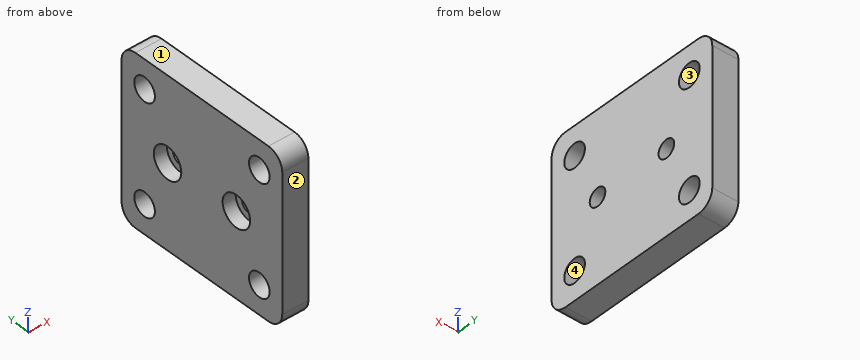
from build123d import *

# Parameters (mm, degrees)
SKETCH_1_W      = 32
SKETCH_1_H      = 35
SKETCH_1_R      = 2.25
SKETCH_1_R_2    = 3
EXTRUDE_1_DEPTH = 2.5
SKETCH_2_W      = 32
SKETCH_2_H      = 35
SKETCH_2_R      = 2.25
SKETCH_2_R_2    = 1.7
EXTRUDE_2_DEPTH = 2.5
FILLET_1_R      = 3


with BuildPart() as part:
    # 草图1 → 凸台-拉伸1 (new body)
    with BuildSketch(Plane(origin=(0, 0, 0), x_dir=(0, 0, -1), z_dir=(1, 0, 0))):
        with Locations((16, 17.5)):
            Rectangle(SKETCH_1_W, SKETCH_1_H)
        with Locations((5.5, 30)):
            Circle(SKETCH_1_R, mode=Mode.SUBTRACT)
        with Locations((26.5, 30)):
            Circle(SKETCH_1_R, mode=Mode.SUBTRACT)
        with Locations((5.5, 5)):
            Circle(SKETCH_1_R, mode=Mode.SUBTRACT)
        with Locations((26.5, 5)):
            Circle(SKETCH_1_R, mode=Mode.SUBTRACT)
        with Locations((16, 25)):
            Circle(SKETCH_1_R_2, mode=Mode.SUBTRACT)
        with Locations((16, 10)):
            Circle(SKETCH_1_R_2, mode=Mode.SUBTRACT)
    extrude(amount=EXTRUDE_1_DEPTH)

    # 草图2 → 凸台-拉伸2 (add)
    with BuildSketch(Plane(origin=(2.5, 0, 0), x_dir=(0, 0, -1), z_dir=(1, 0, 0))):
        with Locations((16, 17.5)):
            Rectangle(SKETCH_2_W, SKETCH_2_H)
        with Locations((26.5, 5)):
            Circle(SKETCH_2_R, mode=Mode.SUBTRACT)
        with Locations((5.5, 5)):
            Circle(SKETCH_2_R, mode=Mode.SUBTRACT)
        with Locations((26.5, 30)):
            Circle(SKETCH_2_R, mode=Mode.SUBTRACT)
        with Locations((5.5, 30)):
            Circle(SKETCH_2_R, mode=Mode.SUBTRACT)
        with Locations((16, 25)):
            Circle(SKETCH_2_R_2, mode=Mode.SUBTRACT)
        with Locations((16, 10)):
            Circle(SKETCH_2_R_2, mode=Mode.SUBTRACT)
    extrude(amount=EXTRUDE_2_DEPTH)

    # 圆角1
    fillet_1_edges = [part.edges().sort_by_distance(p)[0] for p in [
        (2.5, 35, 0),
        (2.5, 35, -32),
        (2.5, 0, -32),
        (2.5, 0, 0),
    ]]
    fillet(fillet_1_edges, radius=FILLET_1_R)


solid = part.part
Verification items for the finished model (mm, model axes). Face numbers are marked on the shaded views. Coordinates: 2 decimals unless noted, no trailing zeros. Loops run counter-clockwise (first coordinate to the right, second up) from the corner with the lowest first, then second, coordinate; pieces in that order, holes last. Notation, with made-up numbers: (16, 33.25) -> (66, 33.25) arc R24 cw to (66, 69.25) -> close; hole circle Ø8 at (33, 9). An arc over 180 degrees is marked (long way). Answer as a JSON object with one key per item and string values. Group by question number.
Item 1: Scan lines: probe 1 along Y at (x, z) = (1.5, -16); probe 2 along Y at (x, z) = (3.8, -16); probe 3 along X at (y, z) = (12, -14). Record each from-to range of solid material in increasing order.
Item 2: Depth check by flat-ended pin: pin 1 (3.5 mm diameter, centred on y = 5, z = -26.5, fed in from -X); pin 2 (3.5 mm diameter, centred on y = 25, z = -16, fed in from -X). Enter the tip coordinate at first touch or a pass-through.
Item 3: Sectioned sample at D-D on x = 1.85. Record the boundary of the cut face in (y, z), plus the area to 3 significant figures.
Item 4: Sectioned sample at A-A on y = 30. Record the boundary of the cut face in (x, z).
Item 5: Sectioned sample at C-C on y = 10. Record the boundary of the cut face in (x, z), plus the area to 4 significant figures.
Item 6: Mould release check, pull along Z, two halves, no side actions. Record for the marked faces 1, 2, 3 and 4: +Z half, -Z half, draft (parallel to the pull), parting line (faces both ways), or undercut.
Item 7: Sectioned sample at B-B on z = -26.5. Record the boundary of the cut face in (x, y).
Evaluation:
{
 "1": {"probe 1": "y = 0 to 7, 13 to 22, 28 to 35", "probe 2": "y = 0 to 8.3, 11.7 to 23.3, 26.7 to 35", "probe 3": "x = 2.5 to 5"},
 "2": {"pin 1": "passes through", "pin 2": "stops at x = 2.5"},
 "3": {"outline": "(0, -29) arc R3 ccw to (3, -32) -> (32, -32) arc R3 ccw to (35, -29) -> (35, -3) arc R3 ccw to (32, 0) -> (3, 0) arc R3 ccw to (0, -3) -> close; hole circle Ø4.5 at (5, -26.5); hole circle Ø4.5 at (5, -5.5); hole circle Ø6 at (10, -16); hole circle Ø6 at (25, -16); hole circle Ø4.5 at (30, -26.5); hole circle Ø4.5 at (30, -5.5)", "area": "992 mm²"},
 "4": {"outline": "(0, -32) -> (5, -32) -> (5, -28.75) -> (0, -28.75) -> close; (0, -24.25) -> (5, -24.25) -> (5, -7.75) -> (0, -7.75) -> close; (0, -3.25) -> (5, -3.25) -> (5, 0) -> (0, 0) -> close"},
 "5": {"outline": "(0, -32) -> (5, -32) -> (5, -17.7) -> (2.5, -17.7) -> (2.5, -19) -> (0, -19) -> close; (0, -13) -> (2.5, -13) -> (2.5, -14.3) -> (5, -14.3) -> (5, 0) -> (0, 0) -> close", "area": "136.5 mm²"},
 "6": {"face 1": "+Z half", "face 2": "draft", "face 3": "undercut", "face 4": "undercut"},
 "7": {"outline": "(0, 0) -> (5, 0) -> (5, 2.75) -> (0, 2.75) -> close; (0, 7.25) -> (5, 7.25) -> (5, 27.75) -> (0, 27.75) -> close; (0, 32.25) -> (5, 32.25) -> (5, 35) -> (0, 35) -> close"}
}
